```python
from build123d import *

# Parameters (mm, degrees)
F1_START = -3
F0_R     = 9.5
F0_R_2   = 6.1
F1_DEPTH = 55
F2_START = -29
F0_R_3   = 15
F2_DEPTH = 3


with BuildPart() as f1:
    # F0 (on Right) → F1 (new body)
    with BuildSketch(Plane.YZ.offset(F1_START)):
        Circle(F0_R)
        Circle(F0_R_2, mode=Mode.SUBTRACT)
    extrude(amount=-F1_DEPTH)

    # F0 (on Right) → F2 (join)
    with BuildSketch(Plane.YZ.offset(F2_START)):
        Circle(F0_R_3)
        Circle(F0_R, mode=Mode.SUBTRACT)
    extrude(amount=-F2_DEPTH)


solid = f1.part
```
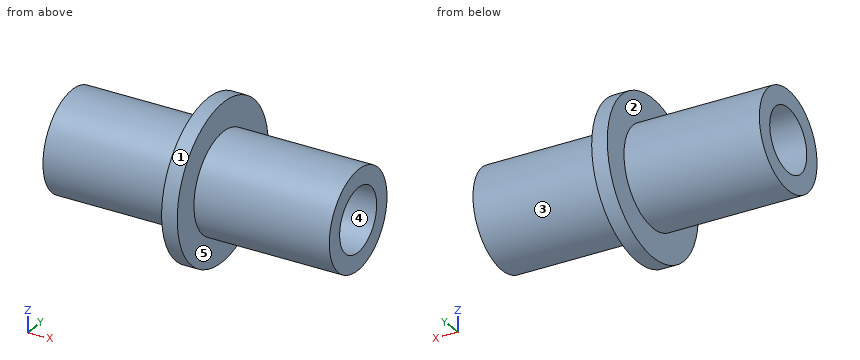
Check sheet for the modelled part. Datum: model origin and axes. Units: mm. Face numbers are marked on the shaded views. A direction names the side the tool comes from. Give positions to 0.01 mm unless a question says otherwise; leave off trailing zeros. Loops run counter-clockwise (first coordinate to the right, second up) from the corner with the lowest first, then second, coordinate; pieces in that order, holes last. Notation, with made-up numbers: (-11, 0.5) - (14, 0.5) arc R23 cw to (14, 39.5) - close; hole circle Ø4 at (69.25, 45). An arc over 180 degrees is marked (long way). One line per question, with ' | ' between items. Start each with the question number.
1. Cross-section at A-A, the plane z = 0. Enter the section's corners in (x, y).
2. Cross-section at C-C, the plane x = -30. Enter the section's corners in (y, z).
3. Set-up check for the marked faces 1 and 2: record each of +Z, -Z, +X, -X, +Y, -Y from which the full face is reachable in a straight line by a thin tool's end or side.
4. Material ranges on line 1 along Z through (x, y) = (-35.5, 0); line 2 along X through (y, z) = (7.75, 10); line 3 along Y through (x, z) = (-48.5, -0.25), recorded low to high. Write a range as [from, to].
5. Cross-section at D-D, the plane y = 8.25. Enter the section's corners in (x, z), plus the area to 3 significant figures.
6. Gauge pin test, flat ends, axial feed: pin 1 Ø1.5 at (x, z) = (-21, -6.5) entering from -Y; pin 2 Ø10 at (y, z) = (0, 0) entering from +X; pin 3 Ø1 at (x, z) = (-51, -7) entering from -Y; pin 4 Ø12 at (y, z) = (3, -11) entering from +X. Record the tip position at first contact, or that the pin passes through.
7. Draft check along Y on the marked faces 3, 4 and 5. Enter one of: released by +Y, released by -Y, zero draft, split by the parting line, or undercut.
Check result:
1) outline: (-58, -9.5) - (-32, -9.5) - (-32, -15) - (-29, -15) - (-29, -9.5) - (-3, -9.5) - (-3, -6.1) - (-58, -6.1) - close; (-58, 6.1) - (-3, 6.1) - (-3, 9.5) - (-29, 9.5) - (-29, 15) - (-32, 15) - (-32, 9.5) - (-58, 9.5) - close
2) outline: circle Ø30 at (0, 0); hole circle Ø12.2 at (0, 0)
3) face 1: +X, -X | face 2: -X
4) line 1: z = [-9.5, -6.1], [6.1, 9.5] | line 2: x = [-32, -29] | line 3: y = [-9.5, -6.09], [6.09, 9.5]
5) outline: (-58, -4.71) - (-32, -4.71) - (-32, -12.53) - (-29, -12.53) - (-29, -4.71) - (-3, -4.71) - (-3, 4.71) - (-29, 4.71) - (-29, 12.53) - (-32, 12.53) - (-32, 4.71) - (-58, 4.71) - close | area: 565 mm2
6) pin 1: stops at y = -7.56 | pin 2: passes through | pin 3: stops at y = -6.93 | pin 4: stops at x = -3
7) face 3: split by the parting line | face 4: undercut | face 5: zero draft
